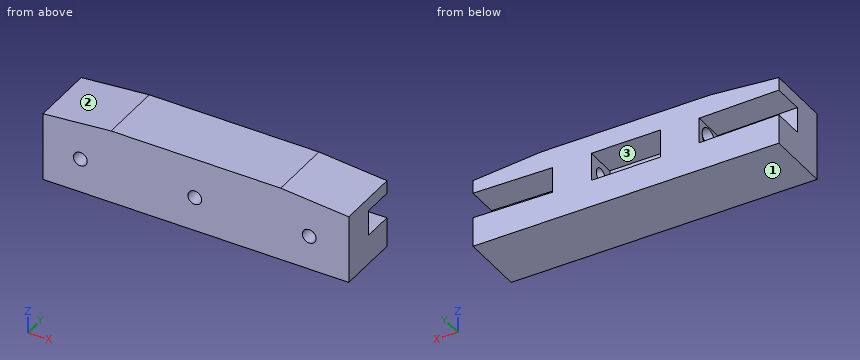
Autodesk Inventor part; units mm, degrees
ref_plane "YZ Plane" through (0, 0, 0) normal (1, 0, 0) x (0, 1, 0)
ref_plane "XZ Plane" through (0, 0, 0) normal (0, 1, 0) x (-1, 0, 0)
ref_plane "XY Plane" through (0, 0, 0) normal (0, 0, 1) x (1, 0, 0)
sketch "Sketch1" plane through (0, 0, 0) normal (0, 1, 0) x (-1, 0, 0)
  line L0 (-10.4458, -2.7323) -> (-10.4458, 5.0177)
  line L1 (-10.4458, 5.0177) -> (9.7542, 5.0177)
  line L2 (9.7542, 5.0177) -> (9.7542, -2.7323)
  line L3 (9.7542, -2.7323) -> (-10.4458, -2.7323)
  line L4 (46.0042, -11.3323) -> (-46.6958, -11.3323)
  line L5 (46.0042, 9.3619) -> (46.0042, -11.3323)
  line L6 (25.3638, 11.1677) -> (46.0042, 9.3619)
  line L7 (-26.0554, 11.1677) -> (25.3638, 11.1677)
  line L8 (-46.6958, 9.3619) -> (-26.0554, 11.1677)
  line L9 (-46.6958, 9.3619) -> (-46.6958, -11.3323)
  line L10 (10.1542, 5.4177) -> (-10.8458, 5.4177)
  line L11 (-10.8458, 5.4177) -> (-10.8458, -3.1323)
  line L12 (-10.8458, -3.1323) -> (10.1542, -3.1323)
  line L13 (10.1542, -3.1323) -> (10.1542, 5.4177)
  line L14 (-10.8458, 5.0177) -> (-22.5458, 5.0177)
  line L15 (-22.5458, 5.0177) -> (-22.5458, -2.7323)
  line L16 (-22.5458, -2.7323) -> (-10.8458, -2.7323)
  line L17 (-0.3458, 5.0177) -> (-0.3458, 1.5521) construction
  line L18 (-22.5458, 5.0177) -> (-46.6958, 5.4177)
  line L19 (-22.5458, -2.7323) -> (-46.6958, -2.3323)
  line L20 (21.8542, 5.0177) -> (46.0042, 5.4177)
  line L21 (21.8542, -2.7323) -> (46.0042, -2.3323)
  line L22 (21.8542, -2.7323) -> (10.1542, -2.7323)
  line L23 (21.8542, 5.0177) -> (21.8542, -2.7323)
  line L24 (10.1542, 5.0177) -> (21.8542, 5.0177)
  point P0 (0, 0)
  dimension "d0" = 0.4
  dimension "d1" = 11.7
extrude "Extrusion1" add sketch "Sketch1" along normal blind 9.398 contours L4 L9 L19 L16 L11 L12 L13 L22 L21 L5 | L20 L24 L13 L10 L11 L14 L18 L9 L8 L7 L6 L5 | L22 L13 L24 L23 | L15 L14 L11 L16
sketch "Sketch2" plane through (0, 0, 0) normal (0, -1, 0) x (1, 0, 0)
  line L0 (-21.8542, 5.0177) -> (-46.0042, 5.4177)
  line L1 (-21.8542, -2.7323) -> (-21.8542, 5.0177)
  line L2 (-46.0042, -2.3323) -> (-21.8542, -2.7323)
  line L3 (-46.0042, -11.3323) -> (-46.0042, -2.3323)
  line L4 (46.6958, -11.3323) -> (-46.0042, -11.3323)
  line L5 (46.6958, -2.3323) -> (46.6958, -11.3323)
  line L6 (22.5458, -2.7323) -> (46.6958, -2.3323)
  line L7 (22.5458, 5.0177) -> (22.5458, -2.7323)
  line L8 (46.6958, 5.4177) -> (22.5458, 5.0177)
  line L9 (46.6958, 9.3619) -> (46.6958, 5.4177)
  line L10 (26.0554, 11.1677) -> (46.6958, 9.3619)
  line L11 (-25.3638, 11.1677) -> (26.0554, 11.1677)
  line L12 (-46.0042, 9.3619) -> (-25.3638, 11.1677)
  line L13 (-46.0042, 5.4177) -> (-46.0042, 9.3619)
  line L14 (-10.1542, 5.4177) -> (-10.1542, -3.1323)
  line L15 (10.8458, 5.4177) -> (-10.1542, 5.4177)
  line L16 (10.8458, -3.1323) -> (10.8458, 5.4177)
  line L17 (-10.1542, -3.1323) -> (10.8458, -3.1323)
  line L18 (46.6958, 5.4177) -> (46.6958, -2.3323)
  line L19 (-46.0042, 5.4177) -> (-46.0042, -2.3323)
  point P0 (0, 0)
extrude "Extrusion2" add sketch "Sketch2" along normal blind 10 contours L1 L2 L19 L0 | L0 L13 L12 L11 L10 L9 L8 L7 L6 L5 L4 L3 L2 L1 | L6 L7 L8 L18 | L15 L16 L17 L14
sketch "Sketch3" plane through (0, -10, 0) normal (0, -1, 0) x (1, 0, 0)
  line L0 (46.6958, 9.3619) -> (26.0554, 11.1677)
  line L1 (26.0554, 11.1677) -> (-25.3638, 11.1677)
  line L2 (-25.3638, 11.1677) -> (-46.0042, 9.3619)
  line L3 (-46.0042, 9.3619) -> (-46.0042, -11.3323)
  line L4 (-46.0042, -11.3323) -> (46.6958, -11.3323)
  line L5 (46.6958, -11.3323) -> (46.6958, 9.3619)
  line L6 (46.6958, -0.9852) -> (-46.0042, -0.9852) construction
  circle A0 centre (34.6958, -0.9852) radius 2.1
  line L7 (0, 0) -> (0, -4.846) construction
  circle A1 centre (-34.6958, -0.9852) radius 2.1
  circle A2 centre (0, -0.9852) radius 2.1
  dimension "d6" = 4.2
  dimension "d7" = 12
  dimension "d10" = 4.2
extrude "Extrusion3" cut sketch "Sketch3" against normal blind 8 contours A0 | A1 | A2
sketch "Sketch4" plane through (22.5458, 9.398, 5.0177) normal (1, 0, 0) x (0, 0, -1)
  circle A0 centre (3.875, -4.85) radius 2.25
  point P0 (5.0177, -9.398)
extrude "Extrusion4" cut sketch "Sketch4" along normal blind 8 and the other way blind 50.0253
sketch "Sketch5" plane through (22.5458, 9.398, 5.0177) normal (1, 0, 0) x (0, 0, -1)
  circle A0 centre (3.875, -4.85) radius 2.25
  line L0 (0, -9.398) -> (7.75, -9.398)
  line L1 (7.75, -9.398) -> (7.75, 0)
  line L2 (0, 0) -> (7.75, 0)
  line L3 (0, -9.398) -> (0, 0)
  circle A1 centre (3.875, -4.85) radius 3.3
  point P0 (5.0177, -9.398)
  dimension "d15" = 6.6
extrude "Extrusion5" cut sketch "Sketch5" against normal blind 3.5 contours A0 | A1
mirror "Mirror1" about plane through (0, 0, 0) normal (1, 0, 0) of "Extrusion5"
properties part number "Camera_Clip"
The listing builds one solid part. Answer for the finished solid, in the listing's coordinates (mm). Face numbers are marked on the shaded views. Round coordinates to 2 decimals unless told otherwise and drop trailing zeros. Order: outer loops, then holes, each group sorted by start corner. A loop starts at its lowest first (then second) coordinate and runs counter-clockwise, first axis right, second up. Notation, with made-up numbers: (-3.5, -11.5) - (53.5, -11.5) arc R30 cw to (53.5, 14.5) - close; hole circle Ø3 at (27.25, 89). An arc over 180 degrees is marked (long way). Put each result on its own line as item: value. Start each with the question number.
(1) Find section A-A (x = 6). Give the vertices of the cut face in (y, z), plus the area to 3 significant figures.
(2) Determine the mould class of the marked faces 1, 2 and 3 for opening direction X: released by +X, released by -X, zero draft, split by the parting line, or undercut.
(3) Straight lines are drawn through the part: probe 1 along X at (y, z) = (2, -1); probe 2 along Z at (x, y) = (-3, 1); probe 3 along X at (y, z) = (-6.25, -2.25). For each, find the intervals that lie inside material, in ascending order. Write a range as from..to.
(4) Find section C-C (x = -11.5). Give the vertices of the cut face in (y, z).
(5) Find section B-B (y = -7.5). Give the vertices of the cut face in (x, z).
(6) Given P1, Ø2.5, axis at x = 0, z = -0.99, coming from the +Y side; P2, Ø2.5, axis at x = -34.7, z = -0.99, coming from the -Y side; P3, Ø5.5, axis at y = 4.5, z = 1, coming from the -X side, each flat-ended and moving along its own axis, determine where each tip first touches the part or whether it passes through.
(7) Find section D-D (x = 40). Give the vertices of the cut face in (y, z), plus the area to 3 significant figures.
Reply:
1. outline: (-10, -11.33) - (9.4, -11.33) - (9.4, -3.13) - (0, -3.13) - (0, 5.42) - (9.4, 5.42) - (9.4, 11.17) - (-10, 11.17) - close
1. area: 356 mm^2
2. face 1: zero draft
2. face 2: released by -X
2. face 3: undercut
3. probe 1: -21.85..-10.15, 10.85..22.55
3. probe 2: -11.33..-3.13, 5.42..11.17
3. probe 3: -46..-36.37, -33.02..-1.68, 1.68..33.02, 36.37..46.7
4. outline: (-10, -11.33) - (9.4, -11.33) - (9.4, 11.17) - (-10, 11.17) - close; hole circle Ø4.5 at (4.55, 1.14)
5. outline: (-46, -11.33) - (46.7, -11.33) - (46.7, 9.36) - (26.06, 11.17) - (-25.36, 11.17) - (-46, 9.36) - close; hole circle Ø4.2 at (-34.7, -0.99); hole circle Ø4.2 at (0, -0.99); hole circle Ø4.2 at (34.7, -0.99)
6. P1: y = 0
6. P2: y = -2
6. P3: x = -19.05
7. outline: (-10, -11.33) - (9.4, -11.33) - (9.4, -2.44) - (0, -2.44) - (0, 5.31) - (9.4, 5.31) - (9.4, 9.95) - (-10, 9.95) - close
7. area: 340 mm^2
